```python
from build123d import *

# Parameters (mm, degrees)
SKETCH_1_W             = 285
SKETCH_1_H             = 200
EXTRUDE_1_DEPTH        = 4
SKETCH_2_R             = 2.1
SKETCH_2_R_2           = 2.6
CUT_EXTRUDE_1_DEPTH    = 5
SKETCH_3_W             = 200
SKETCH_3_H             = 4
EXTRUDE_1002_DEPTH     = 50
SKETCH_4_R             = 8.5
SKETCH_4_W             = 12.5
SKETCH_4_H             = 20
CUT_EXTRUDE_1350_DEPTH = 5
FILLET_1_R             = 10


with BuildPart() as part:
    # 草图1 → 凸台-拉伸1 (new body)
    with BuildSketch(Plane(origin=(0, 0, 0), x_dir=(1, 0, 0), z_dir=(0, 1, 0))):
        Rectangle(SKETCH_1_W, SKETCH_1_H)
    extrude(amount=EXTRUDE_1_DEPTH)

    # 草图2 → 切除-拉伸1 (cut, through all)
    with BuildSketch(Plane(origin=(0, 4, 0), x_dir=(1, 0, 0), z_dir=(0, 1, 0))):
        with Locations((-37.5, 30)):
            Circle(SKETCH_2_R)
        with Locations((37.5, 30)):
            Circle(SKETCH_2_R)
        with Locations((37.5, -45)):
            Circle(SKETCH_2_R)
        with Locations((-37.5, -45)):
            Circle(SKETCH_2_R)
        with Locations((-100, 90)):
            Circle(SKETCH_2_R_2)
        with Locations((100, 90)):
            Circle(SKETCH_2_R_2)
    extrude(amount=-CUT_EXTRUDE_1_DEPTH, mode=Mode.SUBTRACT)

    # 草图3 → Extrude 1002 (add)
    with BuildSketch(Plane.ZY.offset(142.5)):
        with Locations((0, 2)):
            Rectangle(SKETCH_3_W, SKETCH_3_H)
    extrude(amount=EXTRUDE_1002_DEPTH)

    # 草图4 → Cut-Extrude 1350 (cut, through all)
    with BuildSketch(Plane.XZ):
        with Locations((-162.5, 60)):
            Circle(SKETCH_4_R)
        with Locations((-162.5, -60)):
            Rectangle(SKETCH_4_W, SKETCH_4_H)
    extrude(amount=-CUT_EXTRUDE_1350_DEPTH, mode=Mode.SUBTRACT)

    # 圆角1
    fillet_1_edges = [part.edges().sort_by_distance(p)[0] for p in [
        (-192.5, 2, 100),
    ]]
    fillet(fillet_1_edges, radius=FILLET_1_R)


solid = part.part
```
The listing builds one solid part. Answer for the finished solid, in the listing's coordinates (mm). Coordinates: 2 decimals unless noted, no trailing zeros. Loops run counter-clockwise (first coordinate to the right, second up) from the corner with the lowest first, then second, coordinate; pieces in that order, holes last. Notation, with made-up numbers: (89, 20) -> (127, 20) arc R30 ccw to (127, 52) -> close; hole circle Ø10 at (49, 86.5). An arc over 180 degrees is marked (long way). Use one line per item in the form item = value. Start each with the question number.
Item 1: The part is cut by section A-A on z = -53.5. Determine the outline of the cut face in (x, y), then the cut area to 3 significant figures.
Item 2: The part is cut by section B-B on x = -162.5. Determine the outline of the cut face in (y, z).
Item 3: Consider L1, parallel to X at y = 2.65, z = -90; L2, parallel to Z at x = 37.5, y = 0.95; L3, parallel to Z at x = -162.5, y = 2. Determine where each line is inside the solid, lowest interval first. Write a range as [from, to].
Item 4: A flat-ended cylindrical pin translates along its axis: pin 1 Ø4 at (x, z) = (37.5, -30) entering from -Y. Find the tip coordinate at first contact, or state that the pin passes through.
Item 5: The part is cut by section C-C on z = 60. Determine the outline of the cut face in (x, y), then the cut area to 3 significant figures.
Item 6: The mould has two halves that part along Z. Classify faces 1 (the face through (-164.34, 1.97, 51.7)), 2 (the face through (-189.65, 2.03, 96.99)), 3 (the face through (-23, 0, -1)): released by +Z, released by -Z, zero draft, split by the parting line, or undercut.
Answer key:
q1.outline = (-192.5, 0) -> (-168.75, 0) -> (-168.75, 4) -> (-192.5, 4) -> close; (-156.25, 0) -> (142.5, 0) -> (142.5, 4) -> (-156.25, 4) -> close
q1.area = 1,290 mm2
q2.outline = (0, -100) -> (4, -100) -> (4, -70) -> (0, -70) -> close; (0, -50) -> (4, -50) -> (4, 51.5) -> (0, 51.5) -> close; (0, 68.5) -> (4, 68.5) -> (4, 100) -> (0, 100) -> close
q3.L1 = [-192.5, -102.6], [-97.4, 97.4], [102.6, 142.5]
q3.L2 = [-100, -32.1], [-27.9, 42.9], [47.1, 100]
q3.L3 = [-100, -70], [-50, 51.5], [68.5, 100]
q4.pin_1 = through
q5.outline = (-192.5, 0) -> (-171, 0) -> (-171, 4) -> (-192.5, 4) -> close; (-154, 0) -> (142.5, 0) -> (142.5, 4) -> (-154, 4) -> close
q5.area = 1,270 mm2
q6.face_1 = undercut
q6.face_2 = released by +Z
q6.face_3 = zero draft
